Could you check a few things on this model? Use its own coordinates, in mm. A direction names the side the tool comes from. Give positions to 0.01 mm unless a question says otherwise; leave off trailing zeros. Loops run counter-clockwise (first coordinate to the right, second up) from the corner with the lowest first, then second, coordinate; pieces in that order, holes last. Notation, with made-up numbers: (-26.5, 85.25) - (1.5, 85.25) arc R29 ccw to (1.5, 115.25) - close; hole circle Ø5 at (-35, -33). An arc over 180 degrees is marked (long way). One line per item, written item: value. Start each with the question number.
Q1. If we mould it in two halves opening along Z, with no side actions, what happens to faces 4 (the face through (-37.909, 46.596, -167.977)), 5 (the face through (35, 13, 0))? For each: released by +Z, released by -Z, zero draft, split by the parting line, or undercut.
Q2. I'm going to push flat-ended pins straight in: P1, Ø5, axis at x = -19.5, z = 1.5, coming from the +Y side; P2, Ø12, axis at y = 7, z = -104.5, coming from the +X side; P3, Ø3, axis at y = 38, z = 2, coming from the +X side; P4, Ø2, axis at x = -1, z = -119.5, coming from the +Y side (3 decimals). Where does each tip first touch, or does it pass through?
Q3. I want a section at B-B (x = 35). Please give me the cut outline in (y, z) (3 decimals).
Q4. For faces 1 (the face through (20.141, 15, 3)), 2 (the face through (-29, 22, 0)), 3 (the face through (32, 28.761, -168)), which set-ups out of +Z, -Z, +X, -X, +Y, -Y let a thin tool reach every point of the face, with its end or its side?
Q5. I want a section at C-C (x = -23.5). Please give me the cut outline in (y, z) (3 decimals), then the cut area to 3 significant figures.
Q6. I want a section at A-A (y = 44.45). Please give me the cut outline in (x, z), then the cut area to 3 significant figures.
Q7. I want a section at D-D (z = -36). Please give me the cut outline in (x, y) (3 decimals).
Q8. If I drill on line 1 (Y direction, x = -37.5, z = -56) (3 decimals); line 2 (Z direction, x = 22, y = 14), over which ranges is the centre line in solid material (lowest first)? Write a range as from..to.
```python
from build123d import *

# Parameters (mm, degrees)
SKETCH1_R           = 6.35
SKETCH1_R_2         = 4.119285102
SKETCH1_R_3         = 3.175
BOSS_EXTRUDE1_DEPTH = 6.35
SKETCH2_W           = 88.9
SKETCH2_H           = 6.35
BOSS_EXTRUDE2_DEPTH = 177.546
FILLET1_R           = 2.54


with BuildPart() as part:
    # Sketch1 → Boss-Extrude1 (new body)
    with BuildSketch(Plane.XY):
        Polygon((44.45, 28.761098675), (20.141329975, 28.761098675), (20.141329975, 3.175), (-5.261436706, 3.175), (-5.261436706, 25.4), (-26.5176, 25.4), (-26.5176, 50.8), (-44.45, 50.8), (-44.45, 3.175), (-44.45, -3.175), (44.45, -3.175), (44.45, 3.175), align=None)
        with Locations((31.995505277, 19.05)):
            Circle(SKETCH1_R, mode=Mode.SUBTRACT)
        with Locations((-11.602215411, 13.310324548)):
            Circle(SKETCH1_R_2, mode=Mode.SUBTRACT)
        with Locations((-35.568494723, 44.45)):
            Circle(SKETCH1_R_3, mode=Mode.SUBTRACT)
    boss_extrude1 = extrude(amount=BOSS_EXTRUDE1_DEPTH)

    # Sketch2 → Boss-Extrude2 (add)
    with BuildSketch(Plane.XY.offset(6.35)):
        Rectangle(SKETCH2_W, SKETCH2_H)
    extrude(amount=-BOSS_EXTRUDE2_DEPTH)

    # Fillet1
    fillet1_edges = [part.edges().sort_by_distance(p)[0] for p in [
        (44.45, 28.761098675, 3.175),
        (-44.45, 50.8, 3.175),
        (-26.5176, 50.8, 3.175),
        (-5.261436706, 25.4, 3.175),
        (20.141329975, 28.761098675, 3.175),
    ]]
    fillet(fillet1_edges, radius=FILLET1_R)

    # Mirror1: Boss-Extrude1 across plane
    add(boss_extrude1.mirror(Plane.XY.offset(-82.423)))


solid = part.part
```
Worked answers:
1. face 4: zero draft
1. face 5: undercut
2. P1: stops at y = 25.4
2. P2: stops at x = 44.45
2. P3: stops at x = -26.52
2. P4: stops at y = 3.175
3. outline: (-3.175, -171.196) - (13.456, -171.196) - (13.456, -164.846) - (3.175, -164.846) - (3.175, 0) - (13.456, 0) - (13.456, 6.35) - (-3.175, 6.35) - close; (24.644, -171.196) - (28.761, -171.196) - (28.761, -164.846) - (24.644, -164.846) - close; (24.644, 0) - (28.761, 0) - (28.761, 6.35) - (24.644, 6.35) - close
4. face 1: +Z, -Z, +Y
4. face 2: +X, -X, +Y
4. face 3: +Z, -Z, +X, +Y
5. outline: (-3.175, -171.196) - (25.4, -171.196) - (25.4, -164.846) - (3.175, -164.846) - (3.175, 0) - (25.4, 0) - (25.4, 6.35) - (-3.175, 6.35) - close
5. area: 1,410 mm²
6. outline: (-44.45, -171.2) - (-38.74, -171.2) - (-38.74, -164.85) - (-44.45, -164.85) - close; (-44.45, 0) - (-38.74, 0) - (-38.74, 6.35) - (-44.45, 6.35) - close; (-32.39, -171.2) - (-26.52, -171.2) - (-26.52, -164.85) - (-32.39, -164.85) - close; (-32.39, 0) - (-26.52, 0) - (-26.52, 6.35) - (-32.39, 6.35) - close
6. area: 147 mm²
7. outline: (-44.45, -3.175) - (44.45, -3.175) - (44.45, 3.175) - (-44.45, 3.175) - close
8. line 1: y = -3.175..3.175
8. line 2: z = -171.2..-164.85, 0..6.35
